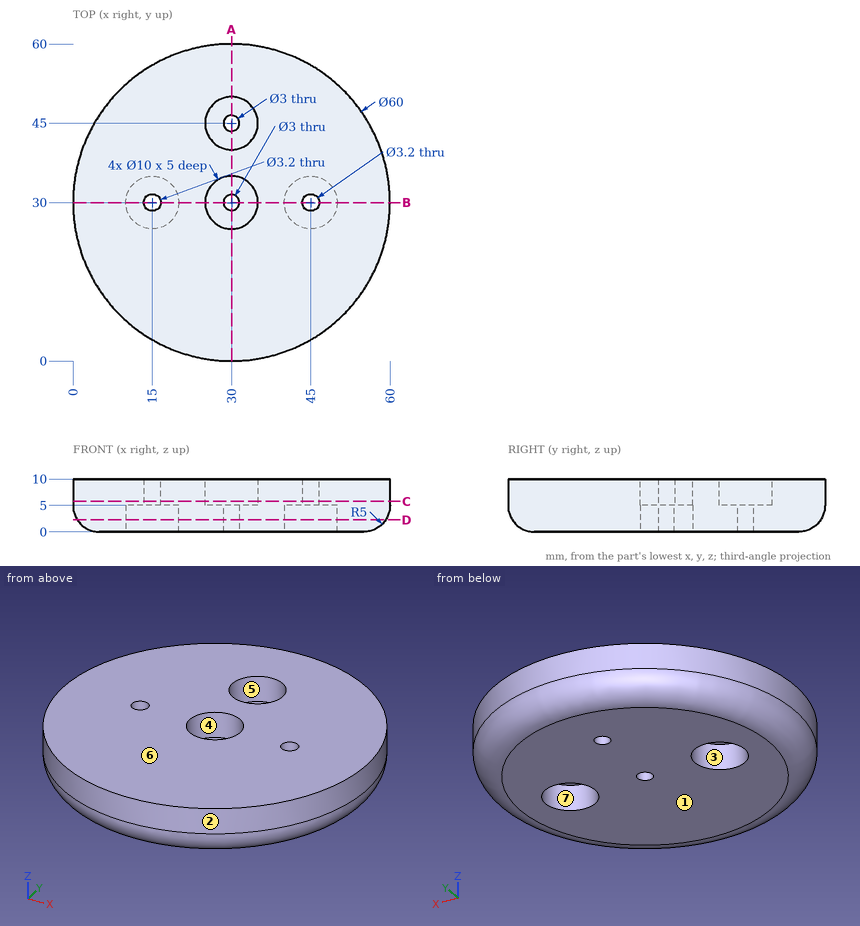
Job drawing, mm, ordinate dimensions from the low corner. One solid piece. A direction names the side the tool comes from. Coordinates: 2 decimals unless noted, no trailing zeros. Order: outer loops, then holes, each group sorted by start corner. A loop starts at its lowest first (then second) coordinate and runs counter-clockwise, first axis right, second up. Notation, with made-up numbers: (25, 14) -> (50, 14) arc R21 ccw to (50, 43) -> close; hole circle Ø6 at (32, 48). An arc over 180 degrees is marked (long way). Return JSON: item names as keys, results as strings. Group by question number.
Item 1: Saw through at C-C on z = 5.75. Write the cut outline in (x, y).
Item 2: Wall check: line 1 along Y through (x, z) = (30, 8.15); line 2 along Y through (x, z) = (30, 1.5); line 3 along Z through (x, y) = (45, 50.5). Give the ranges that are in metal, low to high. Write a range as [from, to].
Item 3: Saw through at A-A on x = 30. Write the cut outline in (y, z), then the cut area to 3 significant figures.
Item 4: Pull direction X, two halves, no side cores. Call the marked faces 1, 2, 3 and 4: pulls with the +X half, pulls with the -X half, needs draft (parallel to the pull), parting line crosses it, or undercut.
Item 5: Flat gauge pins, fed straight in: P1, Ø1.8, axis at x = 30, y = 45, coming from the -Z side; P2, Ø4, axis at x = 17, z = 5, coming from the -Y side; P3, Ø3, axis at x = 17, y = 30.5, coming from the -Z side; P4, Ø4, axis at x = 9.5, z = 7.5, coming from the +Y side. Where does each tip first touch, or does it go through?
Item 6: Saw through at B-B on y = 30. State how many separate pieces and enclosed holes the cut face has, then the cut area to 3 significant figures.
Item 7: Tool access for the marked faces 5, 6 and 7: list every direction of +Z, -Z, +X, -X, +Y, -Y with a clear straight run to the whole face (end or side of a thin tool).
Item 8: Saw through at D-D on z = 2.25. Write the cut outline in (x, y), then the cut area to 3 significant figures.
Values found:
{
 "1": {"outline": "circle Ø60 at (30, 30); hole circle Ø3.2 at (15, 30); hole circle Ø10 at (30, 30); hole circle Ø10 at (30, 45); hole circle Ø3.2 at (45, 30)"},
 "2": {"line 1": "y = [0, 25], [35, 40], [50, 60]", "line 2": "y = [1.43, 28.5], [31.5, 43.5], [46.5, 58.57]", "line 3": "z = [0.02, 10]"},
 "3": {"outline": "(0, 5) arc R5 ccw to (5, 0) -> (28.5, 0) -> (28.5, 5) -> (25, 5) -> (25, 10) -> (0, 10) -> close; (31.5, 0) -> (43.5, 0) -> (43.5, 5) -> (40, 5) -> (40, 10) -> (35, 10) -> (35, 5) -> (31.5, 5) -> close; (46.5, 0) -> (55, 0) arc R5 ccw to (60, 5) -> (60, 10) -> (50, 10) -> (50, 5) -> (46.5, 5) -> close", "area": "459 mm2"},
 "4": {"face 1": "needs draft", "face 2": "parting line crosses it", "face 3": "undercut", "face 4": "undercut"},
 "5": {"P1": "passes through", "P2": "stops at y = 2.09", "P3": "stops at z = 5", "P4": "stops at y = 53.62"},
 "6": {"separate pieces": "4", "enclosed holes": "0", "area": "392 mm2"},
 "7": {"face 5": "+Z", "face 6": "+Z, +X, -X, +Y, -Y", "face 7": "-Z"},
 "8": {"outline": "circle Ø58.35 at (30, 30); hole circle Ø10 at (15, 30); hole circle Ø3 at (30, 30); hole circle Ø3 at (30, 45); hole circle Ø10 at (45, 30)", "area": "2,500 mm2"}
}
